Build history of the part. All positions in model axes, mm. A direction names the side the tool comes from. Give positions to 0.01 mm unless a question says otherwise; leave off trailing zeros. Order: outer loops, then holes, each group sorted by start corner. A loop starts at its lowest first (then second) coordinate and runs counter-clockwise, first axis right, second up. Notation, with made-up numbers: M -24.5,-23.75 L 7.5,-23.75 A16 cw 7.5,1.25 Z; hole C 3.25,-5 d6. An arc over 180 degrees is marked long. Answer as CSV lines item,"result".
from build123d import *

# Parameters (mm, degrees)
F1_ANGLE = 180
F3_DEPTH = 18.5
F4_DEPTH = 8
F6_DEPTH = 18.5
F7_DEPTH = 8
F5_W     = 5
F5_H     = 10
F8_DEPTH = 7
F9_R     = 1


with BuildPart() as f1:
    # F0 (on Top) → F1 (revolve)
    with BuildSketch(Plane.XY):
        Polygon((-9.9, 18.5), (-9.9, 0), (-3.9, 0), (-3.9, 2.5), (-8.1, 11), (-8.1, 16.5), (0, 16.5), (0, 18.5), align=None)
    revolve(axis=Axis((0, -5.2679181099, 0), (0, -1, 0)), revolution_arc=F1_ANGLE)

    # F2 (on face) → F3 (join, through all)
    with BuildSketch(Plane(origin=(0, 18.5, 0), x_dir=(-1, 0, 0), z_dir=(0, 1, 0))):
        with BuildLine():
            ThreePointArc((4.3e-08, -9.9), (-7.0003571186, -7.0003571489), (-9.9, 0))
            Line((-9.9, 0), (-9.9, -9.9))
            Line((-9.9, -9.9), (4.3e-08, -9.9))
        make_face()
        with BuildLine():
            ThreePointArc((9.9, 0), (7.0003571489, -7.0003571186), (4.3e-08, -9.9))
            Line((4.3e-08, -9.9), (9.9, -9.9))
            Line((9.9, -9.9), (9.9, 0))
        make_face()
    extrude(amount=-F3_DEPTH)

    # F4 (add): a face of the model
    f4_faces = [f1.faces().sort_by_distance(p)[0] for p in [
        (-9.6290221411, 9.25, 0),
    ]]
    extrude(f4_faces, amount=F4_DEPTH)

    # F5 (on face) → F6 (join, through all)
    with BuildSketch(Plane(origin=(0, 18.5, 0), x_dir=(-1, 0, 0), z_dir=(0, 1, 0))):
        with BuildLine():
            ThreePointArc((9.9, -5.95), (13.4355339059, -4.4855339059), (14.9, -0.95))
            ThreePointArc((14.9, -0.95), (13.4355339059, 2.5855339059), (9.9, 4.05))
            Line((9.9, 4.05), (9.9, -5.95))
        make_face()
        with BuildLine():
            Line((-9.9, -5.95), (-9.9, 4.05))
            Line((-9.9, 4.05), (-11.9, 4.05))
            ThreePointArc((-11.9, 4.05), (-14.0213203436, 3.1713203436), (-14.9, 1.05))
            Line((-14.9, 1.05), (-14.9, -2.95))
            ThreePointArc((-14.9, -2.95), (-14.0213203436, -5.0713203436), (-11.9, -5.95))
            Line((-11.9, -5.95), (-9.9, -5.95))
        make_face()
    extrude(amount=-F6_DEPTH)

    # F5 (on face) → F7 (cut)
    with BuildSketch(Plane(origin=(0, 18.5, 0), x_dir=(-1, 0, 0), z_dir=(0, 1, 0))):
        with BuildLine():
            ThreePointArc((9.9, -5.95), (13.4355339059, -4.4855339059), (14.9, -0.95))
            ThreePointArc((14.9, -0.95), (13.4355339059, 2.5855339059), (9.9, 4.05))
            Line((9.9, 4.05), (9.9, -5.95))
        make_face()
        with BuildLine():
            Line((-9.9, -5.95), (-9.9, 4.05))
            Line((-9.9, 4.05), (-11.9, 4.05))
            ThreePointArc((-11.9, 4.05), (-14.0213203436, 3.1713203436), (-14.9, 1.05))
            Line((-14.9, 1.05), (-14.9, -2.95))
            ThreePointArc((-14.9, -2.95), (-14.0213203436, -5.0713203436), (-11.9, -5.95))
            Line((-11.9, -5.95), (-9.9, -5.95))
        make_face()
    extrude(amount=-F7_DEPTH, mode=Mode.SUBTRACT)

    # F5 (on face) → F8 (join)
    with BuildSketch(Plane(origin=(0, 18.5, 0), x_dir=(-1, 0, 0), z_dir=(0, 1, 0))):
        with BuildLine():
            Line((9.9, -5.95), (9.9, 4.05))
            ThreePointArc((9.9, 4.05), (4.9, -0.95), (9.9, -5.95))
        make_face()
        with BuildLine():
            ThreePointArc((9.9, -5.95), (4.9, -0.95), (9.9, 4.05))
            Line((9.9, 4.05), (9.9, 8))
            Line((9.9, 8), (-9.9, 8))
            Line((-9.9, 8), (-9.9, 4.05))
            Line((-9.9, 4.05), (-4.9, 4.05))
            Line((-4.9, 4.05), (-4.9, -5.95))
            Line((-4.9, -5.95), (-9.9, -5.95))
            Line((-9.9, -5.95), (-9.9, -9.9))
            Line((-9.9, -9.9), (9.9, -9.9))
            Line((9.9, -9.9), (9.9, -5.95))
        make_face()
        with Locations((-7.4, -0.95)):
            Rectangle(F5_W, F5_H)
    extrude(amount=F8_DEPTH)

    # F9
    f9_edges = [f1.edges().sort_by_distance(p)[0] for p in [
        (9.9, 12.75, 8),
        (-9.9, 12.75, 8),
        (9.9, 12.75, -9.9),
        (-9.9, 12.75, -9.9),
        (-6.9, 0, 8),
        (9.9, 0, 6.025),
        (9.9, 0, -7.925),
        (-9.9, 0, -7.925),
        (-9.9, 0, 6.025),
        (0, 0, -9.9),
        (0, 0, -3.9),
        (-3.9, 0, 4),
        (-14.9, 0, -0.95),
        (10.9, 0, -5.95),
        (14.02132, 0, -5.07132),
        (14.9, 0, -0.95),
        (14.02132, 0, 3.17132),
        (10.9, 0, 4.05),
        (6.9, 0, 8),
        (3.9, 0, 4),
        (0, 25.5, 8),
        (9.9, 25.5, -0.95),
        (0, 25.5, -9.9),
        (-9.9, 25.5, -0.95),
        (14.9, 10.5, -0.95),
        (-14.9, 10.5, -0.95),
        (-3.9, 1.25, 8),
        (-8.1, 11, 4),
        (3.9, 1.25, 8),
        (10.9, 10.5, -5.95),
        (14.02132, 10.5, -5.07132),
        (14.02132, 10.5, 3.17132),
        (10.9, 10.5, 4.05),
        (0, 11, -8.1),
        (8.1, 11, 4),
    ]]
    fillet(f9_edges, radius=F9_R)


solid = f1.part
Item 1: Band-saw the part on B-B (y = 3). Give the cut face in (x, z).
Geometry says:
outline,"M -9.9,-8.9 A1 ccw -8.9,-9.9 L 8.9,-9.9 A1 ccw 9.9,-8.9 L 9.9,-5.95 L 11.9,-5.95 A3 ccw 14.9,-2.95 L 14.9,1.05 A3 ccw 11.9,4.05 L 9.9,4.05 L 9.9,7 A1 ccw 8.9,8 L 4.9,8 A1 ccw 4.15,7.66 L 4.15,0 A4.15 cw -4.15,0 L -4.15,7.66 A1 ccw -4.9,8 L -8.9,8 A1 ccw -9.9,7 L -9.9,4.05 A5 ccw -9.9,-5.95 Z"
Item 2: Probe line 1 along X through (y, z) = (16, 1.5); line 2 along Y through (x, z) = (-8, 5.25); line 3 along Z through (x, y) = (-9, 5.5). List the from-to ranges inside material, lowest first. Write a range as from..to.
Geometry says:
line 1,"x = -9.9..-8.1, 8.1..9.9"
line 2,"y = 0..10.8, 16.5..25.5"
line 3,"z = -9.89..7.99"
Item 3: Drop flat-ended pins along their axis: pin 1 (1.7 mm diameter, centred on y = 1.5, z = 2.5, fed in from +X); pin 2 (2.5 mm diameter, centred on y = 13.5, z = 4, fed in from +X); pin 3 (0.6 mm diameter, centred on x = 11, y = 7, fed in from +Z). Give the stop position or say it passes through.
Geometry says:
pin 1,"stops at x = 14.84"
pin 2,"stops at x = 9.9"
pin 3,"stops at z = 4.05"
Item 4: Band-saw the part on A-A (y = 21.25). Give the cut face in (x, z).
Geometry says:
outline,"M -9.9,-8.9 A1 ccw -8.9,-9.9 L 8.9,-9.9 A1 ccw 9.9,-8.9 L 9.9,7 A1 ccw 8.9,8 L -8.9,8 A1 ccw -9.9,7 Z"
Item 5: Pull direction Y, two halves, no side cores. Call faces 6 (the cylindrical face through (-4.185, 0.301, 3.451)), 7 (the conical face through (-0.12, 5.78, -5.52)), 8 (the flat face through (9.9, 15, -1)): released by +Y, released by -Y, zero draft, split by the parting line, or undercut.
Geometry says:
face 6,"released by -Y"
face 7,"undercut"
face 8,"zero draft"
Item 6: 3-axis set-ups, long thin cutter, end or side, ignore diameter. For faces 1 (the cylindrical face through (10.712, 0.285, -5.649)), 2 (the cylindrical face through (-0.18, 13.9, -8.1)), 3 (the cylindrical face through (10.886, 10.215, -5.649)), 4 (the cylindrical face through (4.3, 2.4, 7.8)), 5 (the cylindrical face through (10.754, 0.285, 3.749)): which of +Z, -Z, +X, -X, +Y, -Y reach the whole face in a straight line?
Geometry says:
face 1,"-Z, +X, -Y"
face 2,"+Z"
face 3,"-Z, +X, +Y"
face 4,"+Z, -Y"
face 5,"+Z, +X, -Y"
